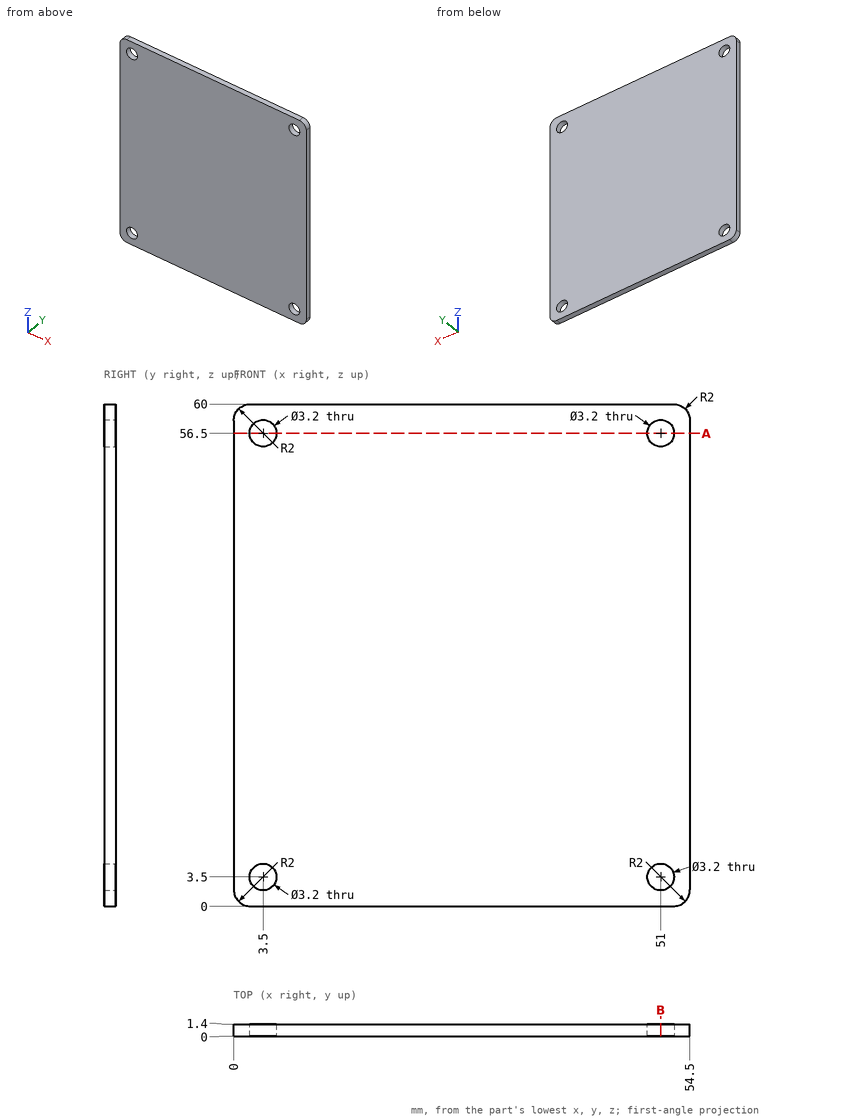
The drawing under review shows one solid part. Ordinate dimensions are in mm from its lowest x, y, z. Give positions to 0.01 mm unless a question says otherwise; leave off trailing zeros. Order: outer loops, then holes, each group sorted by start corner. A loop starts at its lowest first (then second) coordinate and runs counter-clockwise, first axis right, second up. Notation, with made-up numbers: M 38.25,0.5 L 74.25,0.5 A16 cw 74.25,21.5 Z; hole C 11.25,-35 d1. An arc over 180 degrees is marked long. One line per question, with ' | ' between items. Start each with the question number.
Q1. For L1, parallel to Z at x = 3.5, y = 1; L2, parallel to X at y = 0.85, z = 56.5; L3, parallel to Z at x = 50.5, y = 1.05, list the stretches that pass through material, from the lowest coordinate up. Write a range as [from, to].
Q2. We need section B-B (x = 51). Write out the cut boundary in (y, z).
Q3. We need section A-A (z = 56.5). Write out the cut boundary in (x, y).
Returned:
1) L1: [0, 1.9], [5.1, 54.9], [58.1, 60] | L2: [0, 1.9], [5.1, 49.4], [52.6, 54.5] | L3: [0, 1.98], [5.02, 54.98], [58.02, 60]
2) outline: M 0,0 L 1.4,0 L 1.4,1.9 L 0,1.9 Z; M 0,5.1 L 1.4,5.1 L 1.4,54.9 L 0,54.9 Z; M 0,58.1 L 1.4,58.1 L 1.4,60 L 0,60 Z
3) outline: M 0,0 L 1.9,0 L 1.9,1.4 L 0,1.4 Z; M 5.1,0 L 49.4,0 L 49.4,1.4 L 5.1,1.4 Z; M 52.6,0 L 54.5,0 L 54.5,1.4 L 52.6,1.4 Z
